The listing builds one solid part. Answer for the finished solid, in the listing's coordinates (mm). Face numbers are marked on the shaded views. A direction names the side the tool comes from. Round coordinates to 2 decimals unless told otherwise and drop trailing zeros. Answer in a Markdown table with one row per item.
from build123d import *

# Parameters (mm, degrees)
SKETCH1_R           = 3.824529863
BOSS_EXTRUDE1_DEPTH = 8
FILLET1_R           = 3
SKETCH4_R           = 3.824529863
BOSS_EXTRUDE3_DEPTH = 8
SKETCH5_R           = 4
FILLET3_R           = 3


with BuildPart() as part:
    # Sketch1 → Boss-Extrude1 (new body)
    with BuildSketch(Plane(origin=(0, 0, 0), x_dir=(0, 0, -1), z_dir=(1, 0, 0))):
        with BuildLine():
            Line((0, 92), (0, 99))
            Line((0, 99), (-3, 102))
            Line((-3, 102), (-3, 110))
            ThreePointArc((-3, 110), (4.5, 117.5), (12, 110))
            Line((12, 110), (12, 102))
            Line((12, 102), (9, 99))
            Line((9, 99), (9, 92))
            Line((9, 92), (0, 92))
        make_face()
        with Locations((4.5, 110)):
            Circle(SKETCH1_R, mode=Mode.SUBTRACT)
    extrude(amount=BOSS_EXTRUDE1_DEPTH)

    # Fillet1
    fillet1_edges = [part.edges().sort_by_distance(p)[0] for p in [
        (0, 95.5, -9),
        (8, 95.5, 0),
        (8, 95.5, -9),
        (0, 95.5, 0),
    ]]
    fillet(fillet1_edges, radius=FILLET1_R)



with BuildPart() as body_2:
    # Sketch4 → Boss-Extrude3 (new body)
    with BuildSketch(Plane(origin=(30, 0, 0), x_dir=(0, 0, -1), z_dir=(1, 0, 0))):
        with BuildLine():
            Line((-0.004228731, -61.999999953), (8.995771269, -61.999999953))
            Line((8.995771269, -61.999999953), (8.995771269, -68.999999953))
            Line((8.995771269, -68.999999953), (11.995771269, -71.999999953))
            Line((11.995771269, -71.999999953), (11.995771269, -79.999999953))
            ThreePointArc((11.995771269, -79.999999953), (4.495771269, -87.499999953), (-3.004228731, -79.999999953))
            Line((-3.004228731, -79.999999953), (-3.004228731, -71.999999953))
            Line((-3.004228731, -71.999999953), (-0.004228731, -68.999999953))
            Line((-0.004228731, -68.999999953), (-0.004228731, -61.999999953))
        make_face()
        with Locations((4.495771269, -79.999999953)):
            Circle(SKETCH4_R, mode=Mode.SUBTRACT)
    extrude(amount=BOSS_EXTRUDE3_DEPTH)


with BuildPart() as part_1:
    add(part.part)

    add(body_2.part)  # Sweep1 merges body 2
    # Sweep1: sweep along a curve in space
    with BuildLine() as sweep1_path:
        Line((4, 92, -4.5), (4, 86.352130242, -4.5))
        ThreePointArc((4, 86.352130242, -4.5), (5.755444944, 80.69219678, -4.459942659), (10.405301947, 77.019920921, -4.353837987))
        Line((10.405301947, 77.019920921, -4.353837987), (47.364863067, 62.786270522, -3.510461064))
        ThreePointArc((47.364863067, 62.786270522, -3.510461064), (52.019060491, 59.108139902, -3.416609062), (53.77123923, 53.439910597, -3.409333713))
        Line((53.77123923, 53.439910597, -3.409333713), (53.673864596, -23.127444485, -3.913324031))
        ThreePointArc((49.40348763, -33.590655921, -4.071020723), (52.56170451, -28.776861802, -3.973565781), (53.673864596, -23.127444485, -3.913324031))
        Line((38.271359037, -44.984282045, -4.377988717), (49.40348763, -33.590655921, -4.071020723))
        ThreePointArc((34, -55.469085278, -4.495771269), (35.108839506, -49.80804563, -4.465195064), (38.271359037, -44.984282045, -4.377988717))
        Line((34, -61.999999953, -4.495771269), (34, -55.469085278, -4.495771269))
    # Sketch5 → Sweep1 (sweep)
    with BuildSketch(Plane.XZ.offset(-92)):
        with Locations((4, -4.5)):
            Circle(SKETCH5_R)
    sweep(path=sweep1_path.line)

    # Fillet3
    fillet3_edges = [part_1.edges().sort_by_distance(p)[0] for p in [
        (38, -65.499999953, -8.995771269),
        (38, -65.499999953, 0.004228731),
        (30, -65.499999953, -8.995771269),
        (30, -65.499999953, 0.004228731),
    ]]
    fillet(fillet3_edges, radius=FILLET3_R)


solid = part_1.part
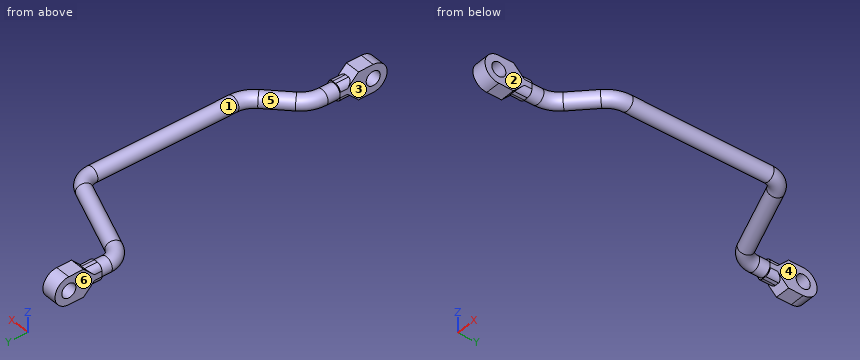
(1) Flat-ended cylindrical pins translate along their axes: pin 1 (9 mm diameter, centred on x = 3, y = 106, fed in from +Z); pin 2 (7.5 mm diameter, centred on y = -77, z = -1, fed in from +X); pin 3 (5 mm diameter, centred on x = 2.5, z = -6.5, fed in from -Y); pin 4 (6 mm diameter, centred on y = 110, z = -4.5, fed in from -X) (3 decimals). Find the tip coordinate at first contact, or state that the pin passes through.
Checked values:
| item | result |
|---|---|
| pin 1 | stops at z = 3 |
| pin 2 | stops at x = 38 |
| pin 3 | stops at y = 76 |
| pin 4 | passes through |
(2) For a pull along Y with two mould halves and no side action, classify the marked faces 5 and 6 as pulls with the +Y half, pulls with the -Y half, needs draft (parallel to the pull), parting line crosses it, or undercut.
Checked values:
| item | result |
|---|---|
| face 5 | undercut |
| face 6 | needs draft |
(3) Find the intervals of material crossed by line 1 (Y direction, x = 33.5, z = -6.25); line 2 (X direction, y = -64.5, z = -6); line 3 (X direction, y = 98, z = -2.5), in increasing order.
Checked values:
| item | result |
|---|---|
| line 1 | y = -87.29 to -83.4, -76.6 to -45.26, 64.74 to 71.56 |
| line 2 | x = 30 to 38 |
| line 3 | x = 0 to 8 |
(4) For the marked faces 1, 2, 3 and 4, determine the directions among +Z, -Z, +X, -X, +Y, -Y from which every point of the face is accessible in a straight line to the end or side of a thin tool.
Checked values:
| item | result |
|---|---|
| face 1 | none |
| face 2 | +Z, -Z, +X, -Y |
| face 3 | +Z, -Z, -X, -Y |
| face 4 | +Z, -Z, +X, +Y |
